```python
from build123d import *

# Parameters (mm, degrees)
SKETCH1_R            = 16.5
SKETCH1_R_2          = 5
BOSS_EXTRUDE1_DEPTH  = 36
SKETCH2_W            = 6
SKETCH2_H            = 6
BOSS_EXTRUDE2_DEPTH  = 1
M3_CLEARANCE_HOLE1_D = 3.4


with BuildPart() as part:
    # Sketch1 → Boss-Extrude1 (new body)
    with BuildSketch(Plane(origin=(0, 0, 0), x_dir=(1, 0, 0), z_dir=(0, 1, 0))):
        with Locations(Location((0, 0, 0), (0, 0, 270))):
            Circle(SKETCH1_R)
        with Locations(Location((0, 0, 0), (0, 0, 270))):
            Circle(SKETCH1_R_2, mode=Mode.SUBTRACT)
    extrude(amount=BOSS_EXTRUDE1_DEPTH)

    # Sketch2 → Boss-Extrude2 (add)
    with BuildSketch(Plane(origin=(0, 36, 0), x_dir=(1, 0, 0), z_dir=(0, 1, 0))):
        with Locations((16.25, 0)):
            Rectangle(SKETCH2_W, SKETCH2_H)
    boss_extrude2 = extrude(amount=BOSS_EXTRUDE2_DEPTH)

    # M3 Clearance Hole1 (through all)
    with Locations(Plane(origin=(0, 37, 0), x_dir=(1, 0, 0), z_dir=(0, 1, 0))):
        with Locations((18.25, 0)):
            m3_clearance_hole1 = Hole(M3_CLEARANCE_HOLE1_D / 2)

    # Mirror1: Boss-Extrude2, M3 Clearance Hole1 across plane
    add(boss_extrude2.mirror(Plane(origin=(0, 0, 0), x_dir=(0, 0, 1), z_dir=(1, 0, 0))))
    add(m3_clearance_hole1.mirror(Plane(origin=(0, 0, 0), x_dir=(0, 0, 1), z_dir=(1, 0, 0))), mode=Mode.SUBTRACT)


solid = part.part
```
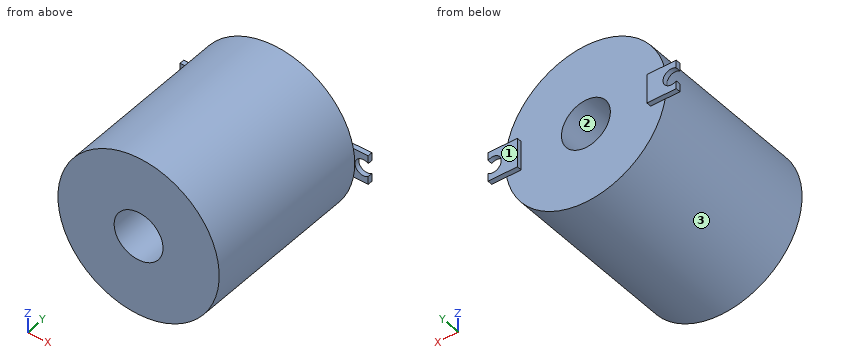
Can you work these out from the model? Positions are in its coordinate system, mm. Face numbers are marked on the shaded views. Round coordinates to 2 decimals unless told otherwise and drop trailing zeros. Order: outer loops, then holes, each group sorted by start corner. A loop starts at its lowest first (then second) coordinate and runs counter-clockwise, first axis right, second up. Notation, with made-up numbers: (-12, 64.5) -> (29, 64.5) arc R16 ccw to (29, 81.5) -> close; hole circle Ø3 at (83.5, 64). An arc over 180 degrees is marked (long way). Return JSON: item names as keys, results as strings. Group by question number.
1. If we section it at C-C, the plane y = 8: Write out the boundary of the cut face in (x, z), then the cut area to 3 significant figures.
2. If we section it at B-B, the plane z = 0: Write out the boundary of the cut face in (x, y), then the cut area to 3 significant figures.
3. We'd pull the mould along X, two halves only. Please class the marked faces 1, 2 and 3: released by +X, released by -X, zero draft, split by the parting line, or undercut.
4. Will these pins go through, and if not, where does the flat tip stop? pin 1 (0.5 mm diameter, centred on x = -17.5, y = 36.5, fed in from +Z); pin 2 (6 mm diameter, centred on x = 15, y = 17, fed in from +Z); pin 3 (12 mm diameter, centred on y = 6, z = -10.5, fed in from +X).
5. If we section it at A-A, the plane x = 18.25: Write out the boundary of the cut face in (y, z).
6. If we section it at D-D, the plane x = 0: Write out the boundary of the cut face in (y, z).
7. I need wall thicknesses on line 1 (Z direction, x = -18.25, y = 36.6); line 2 (X direction, y = 25, z = 0); line 3 (Y direction, x = 11, z = -8.5). Which ranges of each line are inside material? Lowest first, please. Write a range as [from, to].
Output values:
{
 "1": {"outline": "circle Ø33 at (0, 0); hole circle Ø10 at (0, 0)", "area": "777 mm²"},
 "2": {"outline": "(-16.55, 36) -> (-16.5, 36) -> (-16.5, 0) -> (-5, 0) -> (-5, 36) -> (-13.25, 36) -> (-13.25, 37) -> (-16.55, 37) -> close; (5, 0) -> (16.5, 0) -> (16.5, 36) -> (16.55, 36) -> (16.55, 37) -> (13.25, 37) -> (13.25, 36) -> (5, 36) -> close", "area": "835 mm²"},
 "3": {"face 1": "zero draft", "face 2": "undercut", "face 3": "split by the parting line"},
 "4": {"pin 1": "z = 3", "pin 2": "z = 11.32", "pin 3": "x = 15.87"},
 "5": {"outline": "(36, -3) -> (37, -3) -> (37, -1.7) -> (36, -1.7) -> close; (36, 1.7) -> (37, 1.7) -> (37, 3) -> (36, 3) -> close"},
 "6": {"outline": "(0, -16.5) -> (36, -16.5) -> (36, -5) -> (0, -5) -> close; (0, 5) -> (36, 5) -> (36, 16.5) -> (0, 16.5) -> close"},
 "7": {"line 1": "[-3, -1.7], [1.7, 3]", "line 2": "[-16.5, -5], [5, 16.5]", "line 3": "[0, 36]"}
}
